```python
from build123d import *

# Parameters (mm, degrees)
SKETCH1_W           = 17.738061562
SKETCH1_H           = 25.606233094
SKETCH1_R           = 3.175
BOSS_EXTRUDE1_DEPTH = 22.098
SKETCH2_R           = 3.175
BOSS_EXTRUDE2_DEPTH = 5.08
BOSS_EXTRUDE3_REACH = 317.84


with BuildPart() as part:
    # Sketch1 → Boss-Extrude1 (new body)
    with BuildSketch(Plane.XY):
        with Locations((-182.918624156, 225.016931251)):
            Rectangle(SKETCH1_W, SKETCH1_H)
        with Locations(Location((-185.628460018, 223.67720197, 0), (0, 0, 180))):
            Circle(SKETCH1_R, mode=Mode.SUBTRACT)
        with Locations(Location((-186.37244208, 233.67720197, 0), (0, 0, 180))):
            Circle(SKETCH1_R, mode=Mode.SUBTRACT)
    extrude(amount=BOSS_EXTRUDE1_DEPTH)

    # Sketch2 → Boss-Extrude2 (add)
    with BuildSketch(Plane(origin=(-3.393321114, 215.043841855, 6.540236681), x_dir=(0.9998756392437432, 0.015763128213975224, 0.00047941195833239283), z_dir=(-0.01577041682759253, 0.9994135267149823, 0.030395666997209747))):
        Polygon((-199.337975212, -32.034415653), (-170.354814822, 30.120172382), (-150.787629699, 20.995844111), (-179.77079009, -41.158743924), align=None)
        with Locations(Location((-186.334031496, -29.690514452, 0), (0, 0, 270))):
            Circle(SKETCH2_R, mode=Mode.SUBTRACT)
        with Locations(Location((-163.791573415, 18.651942909, 0), (0, 0, 270))):
            Circle(SKETCH2_R, mode=Mode.SUBTRACT)
    extrude(amount=-BOSS_EXTRUDE2_DEPTH)

    # Boss-Extrude3: up to this face of the body (flat: up to its plane)
    boss_extrude3_end = Plane(part.part.faces().sort_by_distance((-182.444308909, 224.507634503, 0))[0])
    # Sketch3 → Boss-Extrude3 (add, up to the picked face)
    with BuildSketch(Plane.XY.offset(22.098), mode=Mode.PRIVATE) as boss_extrude3_sk1:
        Polygon((-191.787654937, 212.213814704), (-191.787654937, 211.652316966), (-174.049593375, 211.933065835), (-174.049593375, 212.213814704), align=None)
    boss_extrude3_tool1 = split(extrude(boss_extrude3_sk1.sketch, amount=-BOSS_EXTRUDE3_REACH, mode=Mode.PRIVATE), bisect_by=boss_extrude3_end, keep=Keep.BOTH, mode=Mode.PRIVATE)
    add(boss_extrude3_tool1.solids().sort_by(Axis((-183.904072, 211.995454, 22.098), (0, 0, -1)))[0])


solid = part.part
```
Geometry: final body of the model. Coordinates: model frame, mm. A direction names the side the tool comes from. Round coordinates to 2 decimals unless told otherwise and drop trailing zeros. Order: outer loops, then holes, each group sorted by start corner. A loop starts at its lowest first (then second) coordinate and runs counter-clockwise, first axis right, second up. Notation, with made-up numbers: (12, 65) - (23, 65) arc R29 cw to (23, 99) - close; hole circle Ø1 at (29, 56). An arc over 180 degrees is marked (long way). Use CSV: the item, a comma, the result in double quotes. Start each with the question number.
Q1. First-contact query: pin 1 (1.5 mm diameter, centred on x = -176, z = -6.5, fed in from -Y); pin 2 (11 mm diameter, centred on y = 227.5, z = 7.5, fed in from -X); pin 3 (8 mm diameter, centred on x = -186, z = 1, fed in from -Y). Flat tips, straight axial feed; report the tip coordinate or a pass-through.
Q2. Access query for faces 1 (the face through (-184.94, 226.777, 10.894)), 2 (the face through (-186.99, 208.69, 37.76)). Directions: +Z, -Z, +X, -X, +Y, -Y. A direction counts if a zero-diameter tool reaches every point of the face in a straight line with its end or side. Return the directions, or none.
Q3. Mould query, pull axis Y, two halves, no side actions, for faces 3 (the face through (-185.684, 236.777, 10.894)), 4 (the face through (-183, 237.82, 11)), 5 (the face through (-181, 225, 22.098)). Classes: +Y half, -Y half, draft (parallel to the pull), parting line (faces both ways), or undercut.
Q4. Section query B-B (y = 222). Return loops of the section in (x, z).
Q5. Section query A-A (z = 14). Return loops of the section in (x, y) (3 decimals), and give its area (3 significant figures).
Q6. Section query C-C (x = -176.5). Return loops of the section in (y, z), and give its area (3 significant figures).
Q7. Material intervals for line 1 along Z through (x, y) = (-179, 231); line 2 along X through (y, z) = (223, 6); line 3 along X through (y, z) = (216, 17.5), sorted ascending. Write a range as from..to.
Q8. Section query D-D (x = -187.5). State how many separate pieces and enclosed holes the cut face has, and give its area (3 significant figures).
Result set:
1,pin 1,"stops at y = 207.61"
1,pin 2,"stops at x = -191.79"
1,pin 3,"stops at y = 207.11"
2,face 1,"+Z, -Z"
2,face 2,"none"
3,face 3,"undercut"
3,face 4,"+Y half"
3,face 5,"draft"
4,outline,"(-191.79, 0) - (-188.32, 0) - (-188.32, 22.1) - (-191.79, 22.1) - close; (-182.93, 0) - (-174.05, 0) - (-174.05, 22.1) - (-182.93, 22.1) - close"
5,outline,"(-191.788, 211.652) - (-191.292, 211.66) - (-191.284, 206.769) - (-167.46, 207.145) - (-167.468, 212.228) - (-174.05, 212.124) - (-174.05, 237.82) - (-191.788, 237.82) - close; hole circle Ø6.35 at (-186.372, 233.677); hole circle Ø6.35 at (-185.628, 223.677)"
5,area,"516 mm2"
6,outline,"(206.41, 33.38) - (207.97, -17.69) - (213.05, -17.7) - (212.51, 0) - (237.82, 0) - (237.82, 22.1) - (211.89, 22.1) - (211.89, 20.28) - (211.5, 33.36) - close"
6,area,"826 mm2"
7,line 1,"z = 0..22.1"
7,line 2,"x = -191.79..-188.73, -182.53..-174.05"
7,line 3,"x = -191.79..-174.05"
8,separate pieces,"4"
8,enclosed holes,"0"
8,area,"507 mm2"
